Solid Edge part; units mm, degrees
sketch "Sketch1" plane through (0, 0, 0) normal (0, 0, 1) x (1, 0, 0)
  line L0 (-10, -9) -> (10, -9)
  line L1 (10, -9) -> (10, 9)
  line L2 (10, 9) -> (-10, 9)
  line L3 (-10, 9) -> (-10, -9)
  dimension "D1" = 10
  dimension "D2" = 10
extrude "Protrusion1" add sketch "Sketch1" along normal blind 15
sketch "Sketch2" plane through (0, 0, 15) normal (0, 0, 1) x (0, 1, 0)
  line L0 (-6.1, 10) -> (6.1, 10)
  line L1 (6.1, 10) -> (6.1, -6)
  line L2 (6.1, -6) -> (-6.1, -6)
  line L3 (-6.1, -6) -> (-6.1, 10)
  dimension "D1" = 6.1
  dimension "D2" = 6.1
extrude "servo_cutout" cut sketch "Sketch2" against normal blind 10
hole "screw_bearing" at (0, 0, 0) direction (0, 0, 1) diameter 4.7 depth 30 tip angle 118 start chamfer 0.6 start chamfer angle 45 end chamfer 0.6 end chamfer angle 45
chamfer "Chamfer1" distance 0.5 angle 45 5 edges at (-2, -6.1, 15) (-10, -6.1, 10) (6, 0, 15) (-2, 6.1, 15) (-10, 6.1, 10)
chamfer "side_chamfer" distance 5 angle 45 1 edges at (10, 0, 0)
sketch "Sketch3" plane through (6, 0, 9.75) normal (-1, 0, 0) x (0, -1, 0)
  line L0 (-6, -2.25) -> (6, -2.25)
  line L1 (6, -2.25) -> (6, 2.75)
  line L2 (6, 2.75) -> (-6, 2.75)
  line L3 (-6, 2.75) -> (-6, -2.25)
  dimension "D1" = 6
  dimension "D2" = 6
extrude "Cutout1" cut sketch "Sketch3" against normal up to next
properties material "Polypropylene, general purpose"
Geometry: final body of the model. Coordinates: model frame, mm. A direction names the side the tool comes from. Round coordinates to 2 decimals unless told otherwise and drop trailing zeros. Order: outer loops, then holes, each group sorted by start corner. A loop starts at its lowest first (then second) coordinate and runs counter-clockwise, first axis right, second up.
Q1. Section C-C, the plane x = 0. Output: boundary loops of the cut face in (y, z).
Result sheet:
outline: (-9, 0) - (-2.95, 0) - (-2.35, 0.6) - (-2.35, 4.4) - (-2.95, 5) - (-6.1, 5) - (-6.1, 14.5) - (-6.6, 15) - (-9, 15) - close; (2.35, 0.6) - (2.95, 0) - (9, 0) - (9, 15) - (6.6, 15) - (6.1, 14.5) - (6.1, 5) - (2.95, 5) - (2.35, 4.4) - close
Q2. Mould query, pull axis X, two halves, no side actions, for faces 4 (the face through (6, 0, 13)), 5 (the face through (2.294, -0.509, 2.527)), 6 (the face through (10, 0, 13)), 7 (the face through (0, -9, 7)). Classes: released by +X, released by -X, zero draft, split by the parting line, or undercut.
Result sheet:
face 4: released by -X
face 5: undercut
face 6: released by +X
face 7: zero draft
Q3. Section A-A, the plane y = 3.75. Output: boundary loops of the cut face in (x, z).
Result sheet:
outline: (-10, 0) - (5, 0) - (10, 5) - (10, 7.5) - (6, 7.5) - (6, 5) - (-10, 5) - close; (6, 12.5) - (10, 12.5) - (10, 15) - (6.5, 15) - (6, 14.5) - close
Q4. Section B-B, the plane y = 0. Output: boundary loops of the cut face in (x, z).
Result sheet:
outline: (-10, 0) - (-2.95, 0) - (-2.35, 0.6) - (-2.35, 4.4) - (-2.95, 5) - (-10, 5) - close; (2.35, 0.6) - (2.95, 0) - (5, 0) - (10, 5) - (10, 7.5) - (6, 7.5) - (6, 5) - (2.95, 5) - (2.35, 4.4) - close; (6, 12.5) - (10, 12.5) - (10, 15) - (6.5, 15) - (6, 14.5) - close
Q5. Material intervals for probe 1 along Y at (x, z) = (-4.75, 10); probe 2 along Y at (x, z) = (7.5, 12); probe 3 along X at (y, z) = (0, 2.5), sorted ascending.
Result sheet:
probe 1: y = -9 to -6.1, 6.1 to 9
probe 2: y = -9 to -6, 6 to 9
probe 3: x = -10 to -2.35, 2.35 to 7.5
Q6. Section D-D, the plane z = 7.75. Output: boundary loops of the cut face in (x, y).
Result sheet:
outline: (-10, -9) - (10, -9) - (10, -6) - (6, -6) - (6, -6.1) - (-9.5, -6.1) - (-10, -6.6) - close; (-10, 6.6) - (-9.5, 6.1) - (6, 6.1) - (6, 6) - (10, 6) - (10, 9) - (-10, 9) - close
Q7. Pin query (flat end, axial travel): pin 1 (1.5 mm diameter, centred on y = 2.5, z = 8.5, fed in from -X); pin 2 (5 mm diameter, centred on y = -1.5, z = 2, fed in from +X); pin 3 (2 mm diameter, centred on x = 8, y = 0, fed in from -Z); pin 4 (8 mm diameter, centred on x = 1.5, y = -1.5, fed in from +Z). Return the tip coordinate at first contact, or that it passes through.
Result sheet:
pin 1: passes through
pin 2: stops at x = 9.5
pin 3: stops at z = 2
pin 4: stops at z = 5
Q8. Access query for faces 1 (the face through (8, -6, 10)), 2 (the face through (-2, -6.1, 10)), 3 (the face through (8, 0, 3)). Directions: +Z, -Z, +X, -X, +Y, -Y. A direction counts if a zero-diameter tool reaches every point of the face in a straight line with its end or side. Return the directions, or none.
Result sheet:
face 1: +X, -X
face 2: +Z, -X
face 3: -Z, +X, +Y, -Y
